Could you check a few things on this model? Use its own coordinates, in mm. A direction names the side the tool comes from. Coordinates: 2 decimals unless noted, no trailing zeros. Loops run counter-clockwise (first coordinate to the right, second up) from the corner with the lowest first, then second, coordinate; pieces in that order, holes last.
1) Will these pins go through, and if not, where does the flat tip stop? P1, Ø4, axis at x = 6.5, y = 10, coming from the -Z side; P2, Ø3, axis at y = 10.5, z = -0.5, coming from the -X side; P3, Ø1, axis at y = 12.5, z = -1.5, coming from the +X side.
2) Thinking about a two-plate mould opening in Y: for faces 1 (the face through (-17, 7.62, -1)), 2 (the face through (1.6, 17.3, 2.086)), 3 (the face through (2, 1.27, -1)), 4 (the face through (2, 20.32, -1)), which applies, released by +Y, released by -Y, zero draft, split by the parting line, or undercut?
3) Imagine slicing it at B-B on y = 15.25. Please give me the cut outline in (x, z).
4) For faces 5 (the face through (-23.414, 4, -1)), 6 (the face through (14.686, 11, -1)), 7 (the face through (-10.714, 11, -1)), which set-ups out of +Z, -Z, +X, -X, +Y, -Y let a thin tool reach every point of the face, with its end or its side?
5) If I drill on line 1 along Y through (x, z) = (-21, 1.25); line 2 along X through (y, z) = (10.5, -2.25); line 3 along Y through (x, z) = (0.5, 1), over which ranges is the centre line in solid material (lowest first)?
6) Imagine slicing it at A-A on x = -16.5. Please give me the cut outline in (y, z), plus the area to 3 significant figures.
7) Imagine slicing it at C-C on z = -0.5. Please give me the cut outline in (x, y) (3 decimals).
```python
from build123d import *

# Parameters (mm, degrees)
SKETCH2_W           = 25.4
SKETCH2_H           = 12.7
BOSS_EXTRUDE1_DEPTH = 21.59
SKETCH3_W           = 12.7
SKETCH3_H           = 7.62
BOSS_EXTRUDE2_DEPTH = 12.7
SKETCH4_R           = 6.35
CUT_EXTRUDE1_DEPTH  = 13.7
SKETCH6_W           = 50.8
SKETCH6_H           = 12.7
CUT_EXTRUDE2_DEPTH  = 1.27
SKETCH7_W           = 50.8
SKETCH7_H           = 12.7
CUT_EXTRUDE3_DEPTH  = 1.27
SKETCH8_W           = 50.8
SKETCH8_H           = 19.05
CUT_EXTRUDE4_DEPTH  = 6.35


with BuildPart() as part:
    # Sketch2 → Boss-Extrude1 (new body)
    with BuildSketch(Plane(origin=(0, 0, 0), x_dir=(1, 0, 0), z_dir=(0, 1, 0))):
        with Locations((1.985818182, -2.085878788)):
            Rectangle(SKETCH2_W, SKETCH2_H)
    extrude(amount=BOSS_EXTRUDE1_DEPTH)

    # Sketch3 → Boss-Extrude2 (add)
    with BuildSketch(Plane.XY.offset(8.435878788)):
        with Locations((-17.064181818, 17.78)):
            Rectangle(SKETCH3_W, SKETCH3_H)
        with Locations((-17.064181818, 3.81)):
            Rectangle(SKETCH3_W, SKETCH3_H)
        with Locations((21.035818182, 17.78)):
            Rectangle(SKETCH3_W, SKETCH3_H)
        with Locations((21.035818182, 3.81)):
            Rectangle(SKETCH3_W, SKETCH3_H)
    extrude(amount=-BOSS_EXTRUDE2_DEPTH)

    # Sketch4 → Cut-Extrude1 (cut, through all)
    with BuildSketch(Plane.XY.offset(8.435878788)):
        with Locations((1.985818182, 10.795)):
            Circle(SKETCH4_R)
    extrude(amount=-CUT_EXTRUDE1_DEPTH, mode=Mode.SUBTRACT)

    # Sketch6 → Cut-Extrude2 (cut)
    with BuildSketch(Plane(origin=(0, 21.59, 0), x_dir=(1, 0, 0), z_dir=(0, 1, 0))):
        with Locations((1.985818182, -2.085878788)):
            Rectangle(SKETCH6_W, SKETCH6_H)
    extrude(amount=-CUT_EXTRUDE2_DEPTH, mode=Mode.SUBTRACT)

    # Sketch7 → Cut-Extrude3 (cut)
    with BuildSketch(Plane.XZ):
        with Locations((1.985818182, 2.085878788)):
            Rectangle(SKETCH7_W, SKETCH7_H)
    extrude(amount=-CUT_EXTRUDE3_DEPTH, mode=Mode.SUBTRACT)

    # Sketch8 → Cut-Extrude4 (cut)
    with BuildSketch(Plane.XY.offset(8.435878788)):
        with Locations((1.985818182, 10.795)):
            Rectangle(SKETCH8_W, SKETCH8_H)
    extrude(amount=-CUT_EXTRUDE4_DEPTH, mode=Mode.SUBTRACT)


solid = part.part
```
Filled in:
1. P1: stops at z = -4.26
1. P2: stops at x = -10.71
1. P3: stops at x = 14.69
2. face 1: undercut
2. face 2: zero draft
2. face 3: released by -Y
2. face 4: released by +Y
3. outline: (-23.41, -4.26) - (-2.54, -4.26) - (-2.54, 2.09) - (-23.41, 2.09) - close; (6.51, -4.26) - (27.39, -4.26) - (27.39, 2.09) - (6.51, 2.09) - close
4. face 5: +Z, -Z, -X, +Y, -Y
4. face 6: +Z, -Z, +X
4. face 7: +Z, -Z, -X
5. line 1: y = 1.27 to 7.62, 13.97 to 20.32
5. line 2: x = -10.71 to -4.36, 8.33 to 14.69
5. line 3: y = 1.27 to 4.62, 16.97 to 20.32
6. outline: (1.27, -4.26) - (7.62, -4.26) - (7.62, 2.09) - (1.27, 2.09) - close; (13.97, -4.26) - (20.32, -4.26) - (20.32, 2.09) - (13.97, 2.09) - close
6. area: 80.6 mm2
7. outline: (-23.414, 1.27) - (27.386, 1.27) - (27.386, 7.62) - (14.686, 7.62) - (14.686, 13.97) - (27.386, 13.97) - (27.386, 20.32) - (-23.414, 20.32) - (-23.414, 13.97) - (-10.714, 13.97) - (-10.714, 7.62) - (-23.414, 7.62) - close; hole circle Ø12.7 at (1.986, 10.795)
